Autodesk Inventor part; units mm, degrees
ref_plane "YZ Plane" through (0, 0, 0) normal (1, 0, 0) x (0, 1, 0)
ref_plane "XZ Plane" through (0, 0, 0) normal (0, 1, 0) x (-1, 0, 0)
ref_plane "XY Plane" through (0, 0, 0) normal (0, 0, 1) x (1, 0, 0)
sketch "Esboço1" plane through (0, 0, 0) normal (0, 0, 1) x (1, 0, 0)
  circle A0 centre (0, 0) radius 2.2
  circle A1 centre (0, 0) radius 4.4
  dimension "d0" = 4.4
  dimension "d1" = 8.8
extrude "Extrusão1" add sketch "Esboço1" along normal blind 0.8
fillet "Arredondamento1" radius 0.1 1 edges at (-4.4, 0, 0.8)
fillet "Arredondamento2" radius 0.1 3 edges at (-2.2, 0, 0.8) (-4.4, 0, 0) (-2.2, 0, 0)
properties part number "Arruela m4" material "Aço inoxidável AISI 304"
Here's how the part is built. I have some questions about the finished solid (model axes, mm). Coordinates: 2 decimals unless noted, no trailing zeros. Write each loop counter-clockwise with the first axis right and the second up, starting at its lowest first coordinate (ties: lowest second). Pieces come first, ordered by that corner, then holes.
1) If I drill on line 1 (Y direction, x = 0, z = 0.45); line 2 (Y direction, x = -0.75, z = 0.65); line 3 (Y direction, x = 3.75, z = 0.15), over which ranges is the centre line in solid material (lowest first)?
Filled in:
line 1: y = -4.4 to -2.2, 2.2 to 4.4
line 2: y = -4.34 to -2.07, 2.07 to 4.34
line 3: y = -2.3 to 2.3
2) If we section it at C-C (z = 0.5): List the corners of the cut face in (x, y) for me.
Filled in:
outline: circle Ø8.8 at (0, 0); hole circle Ø4.4 at (0, 0)
3) If we section it at A-A (x = 0): List the corners of the cut face in (y, z) for me, plus the area to 3 significant figures.
Filled in:
outline: (-4.4, 0.1) arc R0.1 ccw to (-4.3, 0) - (-2.3, 0) arc R0.1 ccw to (-2.2, 0.1) - (-2.2, 0.7) arc R0.1 ccw to (-2.3, 0.8) - (-4.3, 0.8) arc R0.1 ccw to (-4.4, 0.7) - close; (2.2, 0.1) arc R0.1 ccw to (2.3, 0) - (4.3, 0) arc R0.1 ccw to (4.4, 0.1) - (4.4, 0.7) arc R0.1 ccw to (4.3, 0.8) - (2.3, 0.8) arc R0.1 ccw to (2.2, 0.7) - close
area: 3.50 mm2
